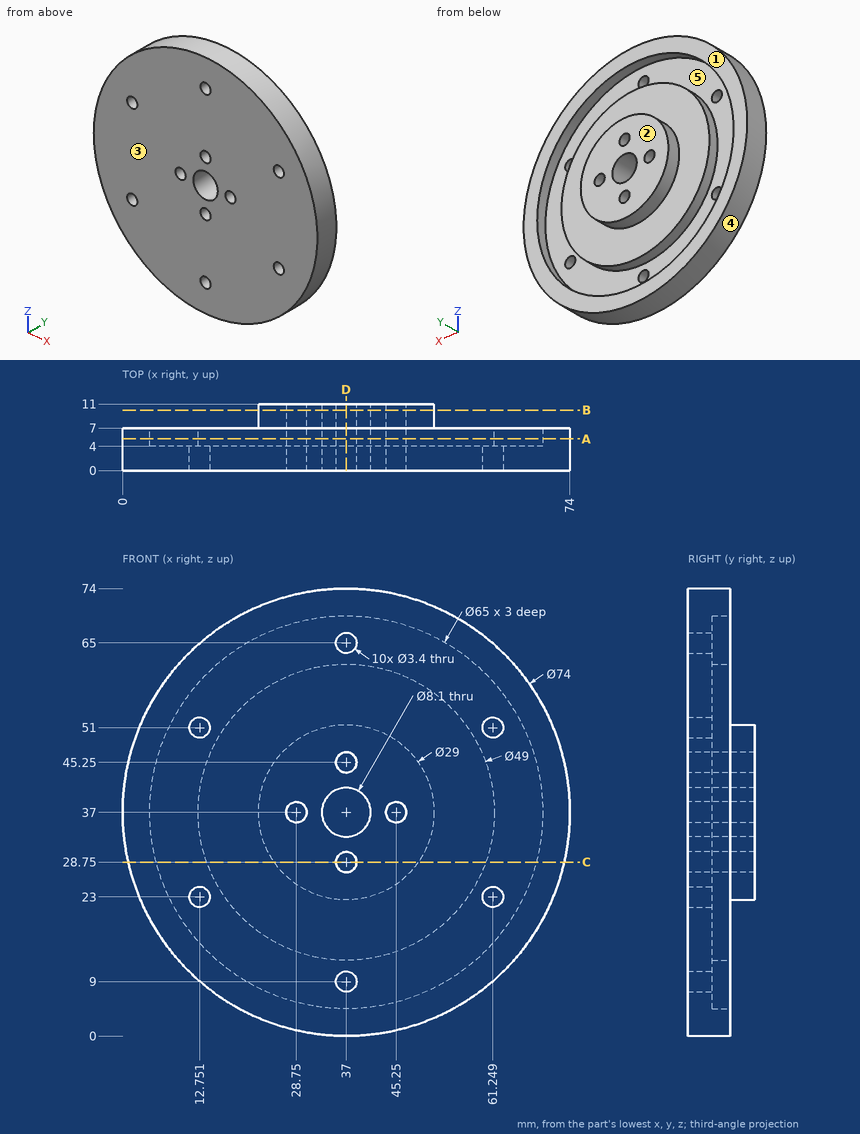
Design review of the part shown in the three views and the two pictorial views. Dimensions are in mm from the part's minimum x, y and z. A direction names the side the tool comes from. Give positions to 0.01 mm unless a question says otherwise; leave off trailing zeros. Order: outer loops, then holes, each group sorted by start corner. A loop starts at its lowest first (then second) coordinate and runs counter-clockwise, first axis right, second up. Notation, with made-up numbers: M -4,47.25 L 18,47.25 A19 cw 18,82.25 Z; hole C 84,18 d3. An arc over 180 degrees is marked long. Answer in a Markdown table with one row per item. Add a question column.
(1) Mouldability with a two-part tool opening along Z and no side actions: class the marked faces 3, 4 and 5 as +Z half, -Z half, draft (parallel to the pull), parting line (faces both ways), or undercut.
(2) Consider section A-A on y = 5.25. State the section outline as (x, z) points.
(3) Wall thickness on probe 1 along X at (y, z) = (4.25, 57); probe 2 along Z at (x, y) = (42, 5.5) (1 decimal); probe 3 along Z at (x, y) = (62, 2.25) (1 decimal): over which ranges is each line inside the solid? List them lowest first. Write a range as [from, to].
(4) For the marked faces 1 and 2, list the 3-axis set-ups (+Z, -Z, +X, -X, +Y, -Y) from which the entire face can be reached by the end or side of a thin tool; tool diameter is ignored.
(5) For pin 1 (4 mm diameter, centred on x = 37, z = 45.25, fed in from +Y); pin 2 (4 mm diameter, centred on x = 46, z = 14.5, fed in from +Y); pin 3 (3 mm diameter, centred on y = 3, z = 57.5, fed in from +X); pin 4 (4 mm diameter, centred on x = 12.75, z = 23, fed in from +Y), all flat-tipped, find the tip position at first contact; note any pin that passes through.
(6) Consider section B-B on y = 10. State the section outline as (x, z) points, and give its area (3 significant figures).
(7) Consider section D-D on x = 37. Give the number of separate pieces and of enclosed holes in the cut face, and give its area (3 significant figures).
(8) Consider section C-C on z = 28.75. State the section outline as (x, y) points (1 decimal), and give its area (3 significant figures).
Evaluation:
| question | item | result |
|---|---|---|
| 1 | face 3 | draft |
| 1 | face 4 | parting line |
| 1 | face 5 | undercut |
| 2 | outline | C 37,37 d74; C 37,37 d49; hole C 37,37 d65; hole C 28.75,37 d3.4; hole C 37,37 d8.1; hole C 37,28.75 d3.4; hole C 37,45.25 d3.4; hole C 45.25,37 d3.4 |
| 3 | probe 1 | x = [5.87, 11.38], [22.85, 51.15], [62.62, 68.13] |
| 3 | probe 2 | z = [0.3, 4.9], [13, 61], [69.1, 73.7] |
| 3 | probe 3 | z = [9.7, 21.5], [24.5, 49.5], [52.5, 64.3] |
| 4 | face 1 | +Y |
| 4 | face 2 | +Z, -Z, +X, -X, +Y |
| 5 | pin 1 | stops at y = 11 |
| 5 | pin 2 | stops at y = 7 |
| 5 | pin 3 | stops at x = 68.75 |
| 5 | pin 4 | stops at y = 4 |
| 6 | outline | C 37,37 d29; hole C 28.75,37 d3.4; hole C 37,37 d8.1; hole C 37,28.75 d3.4; hole C 37,45.25 d3.4; hole C 45.25,37 d3.4 |
| 6 | area | 573 mm^2 |
| 7 | separate pieces | 6 |
| 7 | enclosed holes | 0 |
| 7 | area | 395 mm^2 |
| 8 | outline | M 0.9,0 L 35.3,0 L 35.3,11 L 25.1,11 L 25.1,7 L 13.9,7 L 13.9,4 L 5.6,4 L 5.6,7 L 0.9,7 Z; M 38.7,0 L 73.1,0 L 73.1,7 L 68.4,7 L 68.4,4 L 60.1,4 L 60.1,7 L 48.9,7 L 48.9,11 L 38.7,11 Z |
| 8 | area | 513 mm^2 |
